Could you check a few things on this model? Use its own coordinates, in mm. A direction names the side the tool comes from. Coordinates: 2 decimals unless noted, no trailing zeros. Write each loop counter-clockwise with the first axis right and the second up, starting at its lowest first coordinate (ties: lowest second). Pieces come first, ordered by that corner, then holes. Notation, with made-up numbers: (8, 71.5) - (59, 71.5) arc R17 ccw to (59, 83.5) - close; hole circle Ø9 at (24, 31). An arc over 180 degrees is marked (long way). Answer as a JSON object with one key per item and string values. Group by question number.
1) If we section it at B-B (x = 6.5): Write out the boundary of the cut face in (y, z).
2) If we section it at C-C (z = 19): Write out the boundary of the cut face in (x, y).
3) Will this pin go through, and if not, where does the flat tip stop? pin 1 Ø3.5 at (x, z) = (37.33, 0) entering from +Y.
4) We'd pull the mould along X, two halves only. Please class faces 4 (the flat face through (-50.674, 1, 0)), 5 (the cylindrical face through (-45.82, 4.97, -16.07)), 6 (the flat face through (12.326, 1, 0)): released by +X, released by -X, zero draft, split by the parting line, or undercut.
5) Please list where these lines run through material, in increasing order: line 1 along X through (y, z) = (2.35, 0); line 2 along Z through (x, y) = (9, 2.75); line 3 along X through (y, z) = (1.75, -6).
6) If we section it at A-A (z = 0): Write out the boundary of the cut face in (x, y).
7) If we section it at D-D (y = 4): Write out the boundary of the cut face in (x, z), plus the area to 3 significant figures.
8) On a 3-axis mill with a long thin cutter (end or side, diameter ignored), from which of +Z, -Z, +X, -X, +Y, -Y can I reach the whole of each face in a straight line? I mean faces 1 (the flat face through (-49.688, 1.271, 23.986)), 2 (the cylindrical face through (-45.82, 4.97, 21.93)), 3 (the flat face through (2, 1, -12.5)). Say none if no direction works.
```python
from build123d import *

# Parameters (mm, degrees)
SKETCH1_R                = 1.15
SKETCH1_R_2              = 1.55
BOSS_EXTRUDE1_DEPTH      = 3
BOSS_EXTRUDE1_DEPTH_BACK = 0.506598952
SKETCH2_R                = 3
SKETCH2_R_2              = 1.55
BOSS_EXTRUDE2_DEPTH      = 4


with BuildPart() as part:
    # Sketch1 → Boss-Extrude1 (new body, two sides)
    with BuildSketch(Plane(origin=(0, 0, 0), x_dir=(1, 0, 0), z_dir=(0, 1, 0))) as boss_extrude1_sk:
        Polygon((-48.674262421, -25), (40.325737579, -25), (42.325737579, -23), (42.325737579, 23), (40.325737579, 25), (-48.674262421, 25), (-50.674262421, 23), (-50.674262421, -23), align=None)
        with Locations((37.325737579, 0)):
            Circle(SKETCH1_R, mode=Mode.SUBTRACT)
        with Locations((-45.174262421, 19)):
            Circle(SKETCH1_R_2, mode=Mode.SUBTRACT)
        with Locations((-45.174262421, -19)):
            Circle(SKETCH1_R_2, mode=Mode.SUBTRACT)
        Polygon((-6.674262421, -12.5), (11.325737579, -12.5), (12.325737579, -11.5), (12.325737579, 11.5), (11.325737579, 12.5), (-6.674262421, 12.5), (-7.674262421, 11.5), (-7.674262421, -11.5), align=None, mode=Mode.SUBTRACT)
    extrude(amount=BOSS_EXTRUDE1_DEPTH)
    extrude(boss_extrude1_sk.sketch, amount=-BOSS_EXTRUDE1_DEPTH_BACK)

    # Sketch2 → Boss-Extrude2 (add)
    with BuildSketch(Plane(origin=(0, 3, 0), x_dir=(1, 0, 0), z_dir=(0, 1, 0))):
        with Locations((-45.174262421, 19)):
            Circle(SKETCH2_R)
        with Locations((-45.174262421, 19)):
            Circle(SKETCH2_R_2, mode=Mode.SUBTRACT)
        with Locations((-45.174262421, -19)):
            Circle(SKETCH2_R)
        with Locations((-45.174262421, -19)):
            Circle(SKETCH2_R_2, mode=Mode.SUBTRACT)
    extrude(amount=BOSS_EXTRUDE2_DEPTH)


solid = part.part
```
Here are the results:
{
 "1": {"outline": "(-0.51, -25) - (3, -25) - (3, -12.5) - (-0.51, -12.5) - close; (-0.51, 12.5) - (3, 12.5) - (3, 25) - (-0.51, 25) - close"},
 "2": {"outline": "(-50.67, -0.51) - (-46.72, -0.51) - (-46.72, 7) - (-48.17, 7) - (-48.17, 3) - (-50.67, 3) - close; (-43.62, -0.51) - (42.33, -0.51) - (42.33, 3) - (-42.17, 3) - (-42.17, 7) - (-43.62, 7) - close"},
 "3": {"pin 1": "stops at y = 3"},
 "4": {"face 4": "released by -X", "face 5": "split by the parting line", "face 6": "undercut"},
 "5": {"line 1": "x = -50.67 to -7.67, 12.33 to 36.18, 38.48 to 42.33", "line 2": "z = -25 to -12.5, 12.5 to 25", "line 3": "x = -50.67 to -7.67, 12.33 to 42.33"},
 "6": {"outline": "(-50.67, -0.51) - (-7.67, -0.51) - (-7.67, 3) - (-50.67, 3) - close; (12.33, -0.51) - (36.18, -0.51) - (36.18, 3) - (12.33, 3) - close; (38.48, -0.51) - (42.33, -0.51) - (42.33, 3) - (38.48, 3) - close"},
 "7": {"outline": "circle Ø6 at (-45.17, -19); circle Ø6 at (-45.17, 19); hole circle Ø3.1 at (-45.17, -19); hole circle Ø3.1 at (-45.17, 19)", "area": "41.5 mm²"},
 "8": {"face 1": "+Z, -X, +Y, -Y", "face 2": "+Y", "face 3": "+Y, -Y"}
}
